Here's the drawing with two shaded views (mm, measured from the low corner). I have some questions. A direction names the side the tool comes from. Give positions to 0.01 mm unless a question says otherwise; leave off trailing zeros. Write each loop counter-clockwise with the first axis right and the second up, starting at its lowest first coordinate (ties: lowest second). Pieces come first, ordered by that corner, then holes. Notation, with made-up numbers: (72.25, 76) - (93.25, 76) arc R19 cw to (93.25, 84) - close; hole circle Ø8 at (14.25, 24). An arc over 180 degrees is marked (long way). Use one line per item in the form item = value. Start each with the question number.
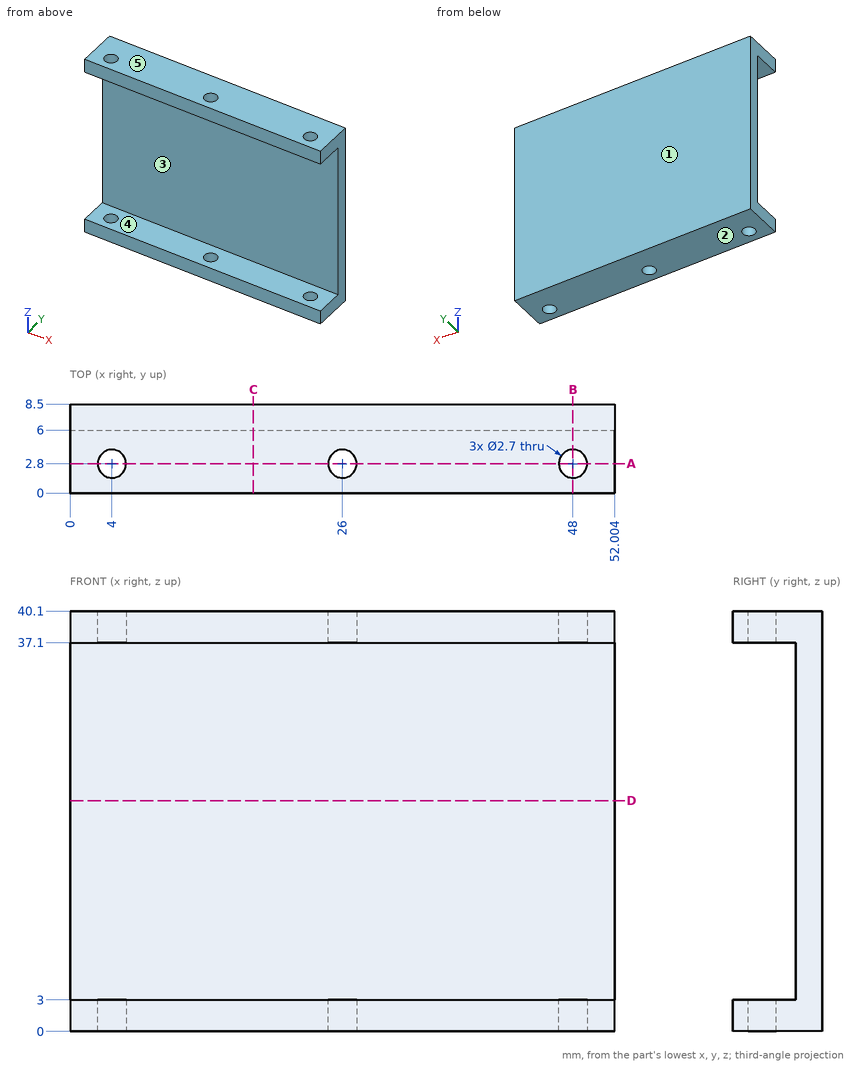
1. I want a section at A-A, the plane y = 2.8. Give the number of separate pieces and of enclosed holes in the cut face, then the cut area to 3 significant figures.
2. Please list where these lines run through material, in increasing order: line 1 (Y direction, x = 4, z = 38.6); line 2 (Z direction, x = 22.5, y = 0.5); line 3 (Y direction, x = 18.5, z = 30.5).
3. I want a section at D-D, the plane z = 22. List the corners of the cut face in (x, y) for me, then the cut area to 3 significant figures.
4. I want a section at C-C, the plane x = 17.5. List the corners of the cut face in (y, z) for me, then the cut area to 3 significant figures.
5. We'd pull the mould along Z, two halves only. Please class the marked faces 1, 2 and 3: pulls with the +Z half, pulls with the -Z half, needs draft (parallel to the pull), parting line crosses it, or undercut.
6. For P1, Ø1.6, axis at x = 4, y = 2.8, coming from the -Z side; P2, Ø1, axis at x = 22, z = 18, coming from the -Y side, each with a flat end and sliding along its axis, tell me the tip position at first contact or that it passes through.
7. I want a section at B-B, the plane x = 48. List the corners of the cut face in (y, z) for me.
8. For the marked faces 4 and 5, which set-ups out of +Z, -Z, +X, -X, +Y, -Y let a thin tool reach every point of the face, with its end or its side?
Result sheet:
q1.separate_pieces = 8
q1.enclosed_holes = 0
q1.area = 263 mm2
q2.line_1 = 0 to 1.45, 4.15 to 8.5
q2.line_2 = 0 to 3, 37.1 to 40.1
q2.line_3 = 6 to 8.5
q3.outline = (0, 6) - (52, 6) - (52, 8.5) - (0, 8.5) - close
q3.area = 130 mm2
q4.outline = (0, 0) - (8.5, 0) - (8.5, 40.1) - (0, 40.1) - (0, 37.1) - (6, 37.1) - (6, 3) - (0, 3) - close
q4.area = 136 mm2
q5.face_1 = needs draft
q5.face_2 = pulls with the -Z half
q5.face_3 = undercut
q6.P1 = through
q6.P2 = 6
q7.outline = (0, 0) - (1.45, 0) - (1.45, 3) - (0, 3) - close; (0, 37.1) - (1.45, 37.1) - (1.45, 40.1) - (0, 40.1) - close; (4.15, 0) - (8.5, 0) - (8.5, 40.1) - (4.15, 40.1) - (4.15, 37.1) - (6, 37.1) - (6, 3) - (4.15, 3) - close
q8.face_4 = +X, -X, -Y
q8.face_5 = +Z, +X, -X, +Y, -Y
